Verification items for the finished model (mm, model axes). Face numbers are marked on the shaded views. A direction names the side the tool comes from. Round coordinates to 2 decimals unless told otherwise and drop trailing zeros. Order: outer loops, then holes, each group sorted by start corner. A loop starts at its lowest first (then second) coordinate and runs counter-clockwise, first axis right, second up. Notation, with made-up numbers: M -26.5,7.5 L 19.5,7.5 A19 ccw 19.5,31.5 Z; hole C 80.5,-27.5 d6. An arc over 180 degrees is marked long. One line per item, written item: value. Start each with the question number.
from build123d import *

# Parameters (mm, degrees)
F0_R     = 7.62
F0_R_2   = 2.3495
F1_DEPTH = 98.171
F2_DEPTH = 18.288
F3_DEPTH = 28.575
F5_DEPTH = 4.445
F7_DEPTH = 10.6045
F8_R     = 2.2225
F9_DEPTH = 2.54


with BuildPart() as f1:
    # F0 (on Top) → F1 (new body)
    with BuildSketch(Plane.XY):
        with BuildLine():
            ThreePointArc((32.0675, 9.017), (30.207628, 13.507128), (25.7175, 15.367))
            Line((25.7175, 15.367), (-25.7175, 15.367))
            ThreePointArc((-25.7175, 15.367), (-30.207628, 13.507128), (-32.0675, 9.017))
            Line((-32.0675, 9.017), (-32.0675, -9.017))
            ThreePointArc((-32.0675, -9.017), (-30.207628, -13.507128), (-25.7175, -15.367))
            Line((-25.7175, -15.367), (25.7175, -15.367))
            ThreePointArc((25.7175, -15.367), (30.207628, -13.507128), (32.0675, -9.017))
            Line((32.0675, -9.017), (32.0675, 9.017))
        make_face()
        with Locations((-13.97, 0)):
            Circle(F0_R, mode=Mode.SUBTRACT)
        with Locations((13.97, 0)):
            Circle(F0_R, mode=Mode.SUBTRACT)
        with Locations((-13.97, 0)):
            Circle(F0_R)
        with Locations((-13.97, 0)):
            Circle(F0_R_2, mode=Mode.SUBTRACT)
        with Locations((-13.97, 0)):
            Circle(F0_R_2)
        with Locations((13.97, 0)):
            Circle(F0_R)
        with Locations((13.97, 0)):
            Circle(F0_R_2, mode=Mode.SUBTRACT)
        with Locations((13.97, 0)):
            Circle(F0_R_2)
    extrude(amount=-F1_DEPTH)

    # F0 (on Top) → F2 (join)
    with BuildSketch(Plane.XY):
        with Locations((-13.97, 0)):
            Circle(F0_R)
        with Locations((-13.97, 0)):
            Circle(F0_R_2, mode=Mode.SUBTRACT)
        with Locations((-13.97, 0)):
            Circle(F0_R_2)
        with Locations((13.97, 0)):
            Circle(F0_R)
        with Locations((13.97, 0)):
            Circle(F0_R_2, mode=Mode.SUBTRACT)
        with Locations((13.97, 0)):
            Circle(F0_R_2)
    extrude(amount=F2_DEPTH)

    # F0 (on Top) → F3 (join)
    with BuildSketch(Plane.XY):
        with Locations((-13.97, 0)):
            Circle(F0_R_2)
        with Locations((13.97, 0)):
            Circle(F0_R_2)
    extrude(amount=F3_DEPTH)

    # F4 (on face) → F5 (cut)
    with BuildSketch(Plane(origin=(0, 0, -98.171), x_dir=(1, 0, 0), z_dir=(0, 0, -1))):
        with BuildLine():
            Line((25.0825, 14.097), (-25.0825, 14.097))
            ThreePointArc((-25.0825, 14.097), (-29.123615, 12.423115), (-30.7975, 8.382))
            Line((-30.7975, 8.382), (-30.7975, -8.382))
            ThreePointArc((-30.7975, -8.382), (-29.123615, -12.423115), (-25.0825, -14.097))
            Line((-25.0825, -14.097), (25.0825, -14.097))
            ThreePointArc((25.0825, -14.097), (29.123615, -12.423115), (30.7975, -8.382))
            Line((30.7975, -8.382), (30.7975, 8.382))
            ThreePointArc((30.7975, 8.382), (29.123615, 12.423115), (25.0825, 14.097))
        make_face()
    extrude(amount=-F5_DEPTH, mode=Mode.SUBTRACT)

    # F6 (on Front) → F7 (join, symmetric)
    with BuildSketch(Plane.XZ):
        with BuildLine():
            ThreePointArc((-29.845, -96.764594), (-31.4325, -98.352094), (-33.02, -96.764594))
            Line((-33.02, -96.764594), (-33.02, -5.715))
            ThreePointArc((-33.02, -5.715), (-33.763949, -3.918949), (-35.56, -3.175))
            Line((-35.56, -3.175), (-44.958, -3.175))
            Line((-44.958, -3.175), (-44.958, -4.826))
            Line((-44.958, -4.826), (-35.941, -4.826))
            ThreePointArc((-35.941, -4.826), (-35.042974, -5.197974), (-34.671, -6.096))
            Line((-34.671, -6.096), (-34.671, -96.764594))
            ThreePointArc((-34.671, -96.764594), (-31.4325, -100.003094), (-28.194, -96.764594))
            Line((-28.194, -96.764594), (-29.845, -96.764594))
        make_face()
        with BuildLine():
            ThreePointArc((33.02, -96.764594), (31.4325, -98.352094), (29.845, -96.764594))
            Line((29.845, -96.764594), (28.194, -96.764594))
            ThreePointArc((28.194, -96.764594), (31.4325, -100.003094), (34.671, -96.764594))
            Line((34.671, -96.764594), (34.671, -6.096))
            ThreePointArc((34.671, -6.096), (35.042974, -5.197974), (35.941, -4.826))
            Line((35.941, -4.826), (44.958, -4.826))
            Line((44.958, -4.826), (44.958, -3.175))
            Line((44.958, -3.175), (35.56, -3.175))
            ThreePointArc((35.56, -3.175), (33.763949, -3.918949), (33.02, -5.715))
            Line((33.02, -5.715), (33.02, -96.764594))
        make_face()
    extrude(amount=F7_DEPTH, both=True)

    # F8 (on face) → F9 (cut)
    with BuildSketch(Plane.XY.offset(-3.175)):
        with Locations((38.1, 0)):
            Circle(F8_R)
        with Locations((-38.1, 0)):
            Circle(F8_R)
    extrude(amount=-F9_DEPTH, mode=Mode.SUBTRACT)


solid = f1.part
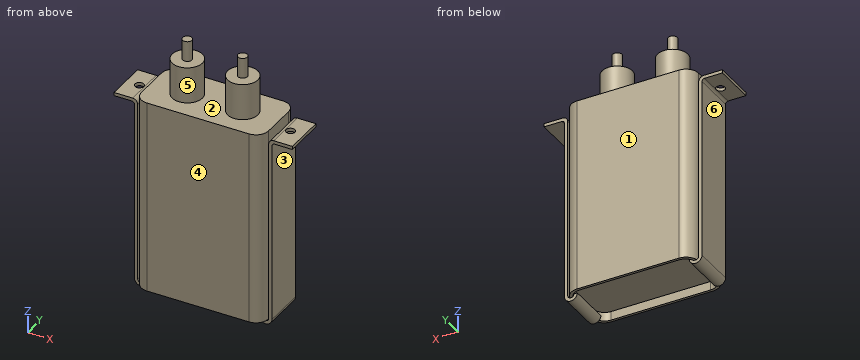
1. Section check C-C (x = 13.97). Record the cut outline in (y, z) (1 decimal).
2. Tool access check on the marked faces 1, 2 and 3. Record the directions out of +Z, -Z, +X, -X, +Y, -Y that give a thin tool (end or side, any length) a straight path to the whole face; none if there is none.
3. Draft check along X on the marked faces 4, 5 and 6. Enter one of: released by +X, released by -X, zero draft, split by the parting line, or undercut.
4. Section check A-A (z = -44.5). Record the cut outline in (x, y).
5. Section check B-B (x = 38.1). Record the cut outline in (y, z) (1 decimal), and give its area (3 significant figures).
6. Section check D-D (z = 16). Record the cut outline in (x, y).
7. Scan lines: line 1 along X through (y, z) = (-6, -7.5); line 2 along Y through (x, z) = (-38.1, -3.6); line 3 along X through (y, z) = (-10.5, -64). Record each from-to range of solid material in increasing order.
8. Depth check by flat-ended pin: pin 1 (17 mm diameter, centred on y = -4.5, z = -71.5, fed in from -X); pin 2 (2.5 mm diameter, centred on x = 38.1, y = 0, fed in from +Z); pin 3 (1.5 mm diameter, centred on y = 11.5, z = -18, fed in from +X); pin 4 (3 mm diameter, centred on x = 25, y = 9.5, fed in from -Z). Enter the tip coordinate at first touch or a pass-through.
Geometry check:
1. outline: M -15.4,-98.2 L -14.1,-98.2 L -14.1,-93.7 L 14.1,-93.7 L 14.1,-98.2 L 15.4,-98.2 L 15.4,0 L 7.6,0 L 7.6,18.3 L 2.3,18.3 L 2.3,28.6 L -2.3,28.6 L -2.3,18.3 L -7.6,18.3 L -7.6,0 L -15.4,0 Z
2. face 1: +Z, -Z, +X, -X, +Y
2. face 2: +Z
2. face 3: -Z, +X, +Y, -Y
3. face 4: zero draft
3. face 5: undercut
3. face 6: released by -X
4. outline: M -34.67,-10.6 L -33.02,-10.6 L -33.02,10.6 L -34.67,10.6 Z; M -32.07,-9.02 A6.35 ccw -25.72,-15.37 L 25.72,-15.37 A6.35 ccw 32.07,-9.02 L 32.07,9.02 A6.35 ccw 25.72,15.37 L -25.72,15.37 A6.35 ccw -32.07,9.02 Z; M 33.02,-10.6 L 34.67,-10.6 L 34.67,10.6 L 33.02,10.6 Z
5. outline: M -10.6,-4.8 L -2.2,-4.8 L -2.2,-3.2 L -10.6,-3.2 Z; M 2.2,-4.8 L 10.6,-4.8 L 10.6,-3.2 L 2.2,-3.2 Z
5. area: 27.7 mm²
6. outline: C -13.97,0 d15.24; C 13.97,0 d15.24
7. line 1: x = -34.67 to -33.02, -32.07 to 32.07, 33.02 to 34.67
7. line 2: y = -10.6 to -2.22, 2.22 to 10.6
7. line 3: x = -34.67 to -33.02, -31.89 to 31.89, 33.02 to 34.67
8. pin 1: stops at x = -34.67
8. pin 2: passes through
8. pin 3: stops at x = 31.83
8. pin 4: stops at z = -93.73
